Could you check a few things on this model? Use its own coordinates, in mm. Give positions to 0.01 mm unless a question says otherwise; leave off trailing zeros. Write each loop counter-clockwise with the first axis right and the second up, starting at its lowest first coordinate (ties: lowest second). Pieces come first, ordered by that corner, then holes. Notation, with made-up numbers: (34.5, 84.5) - (48.5, 84.5) arc R23 cw to (48.5, 109.5) - close; hole circle Ø7 at (-21, -4). An arc over 180 degrees is marked (long way). Answer as CSV lines item,"result". Start each with the question number.
Q1. Will these pins go through, and if not, where does the flat tip stop? pin 1 Ø2 at (x, z) = (15.5, -5) entering from -Y; pin 2 Ø1 at (x, y) = (35, 2) entering from +Z.
Q2. Imagine slicing it at D-D on z = 0. List the corners of the cut face in (x, y) for me, and give its area (3 significant figures).
Q3. Imagine slicing it at B-B on z = -19. List the corners of the cut face in (x, y) for me, and give its area (3 significant figures).
Q4. Imagine slicing it at A-A on y = 1.8. List the corners of the cut face in (x, z) for me, and give its area (3 significant figures).
Q5. If I drill on line 1 along X through (y, z) = (2.4, -19); line 2 along Z through (x, y) = (-9, 3.45); line 3 along Z through (x, y) = (-40, 2.45), over which ranges is the centre line in solid material (lowest first)?
Q6. Imagine slicing it at C-C on x = -40. List the corners of the cut face in (y, z) for me, and give its area (3 significant figures).
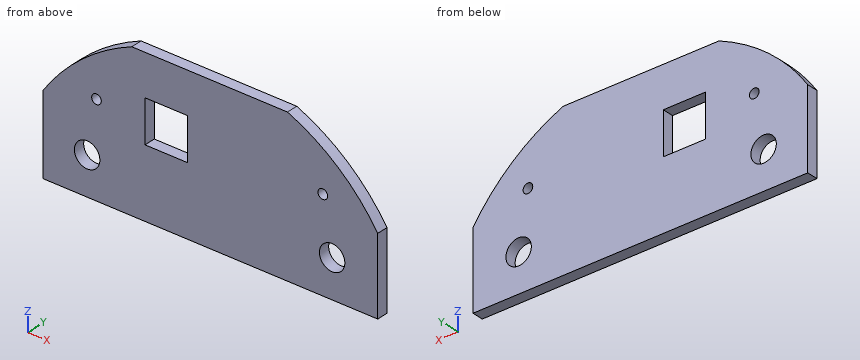
```python
from build123d import *

# Parameters (mm, degrees)
ESQUISSE1_W             = 63
ESQUISSE1_H             = 25
BOSS_EXTRU_1_DEPTH      = 4
D_GAGEMENT_M81_D        = 9
ESQUISSE5_R             = 96
ESQUISSE5_R_2           = 71
ENL_V_MAT_EXTRU_1_DEPTH = 68.845644546
ESQUISSE6_W             = 63
ESQUISSE6_H             = 25
BOSS_EXTRU_2_DEPTH      = 4
ESQUISSE7_W             = 15
ESQUISSE7_H             = 15
ENL_V_MAT_EXTRU_2_DEPTH = 68.845644546
D_GAGEMENT_M31_D        = 3.4


with BuildPart() as part:
    # Esquisse1 → Boss.-Extru.1 (new body)
    with BuildSketch(Plane(origin=(0, 0, 0), x_dir=(1, 0, 0), z_dir=(0, 1, 0))):
        Polygon((-58.901607841, 6.711500167), (-58.901607841, 32.486170288), (59.427941441, 32.486170288), (59.427941441, 7.487213227), (59.427941441, -21.450828615), (-58.901607841, -21.450828615), align=None)
        Rectangle(ESQUISSE1_W, ESQUISSE1_H, mode=Mode.SUBTRACT)
    extrude(amount=BOSS_EXTRU_1_DEPTH)

    # Dégagement M81 (through all)
    with Locations(Plane(origin=(0, 4, 0), x_dir=(1, 0, 0), z_dir=(0, 1, 0))):
        with Locations((-43.3, 19), (43.3, 19)):
            Hole(D_GAGEMENT_M81_D / 2)

    # Esquisse5 → Enlèv. mat.-Extru.1 (cut, through all)
    with BuildSketch(Plane(origin=(0, 4, 0), x_dir=(1, 0, 0), z_dir=(0, 1, 0))):
        with Locations((0, 44.002199903)):
            Circle(ESQUISSE5_R)
        with Locations((0, 44.002199903)):
            Circle(ESQUISSE5_R_2, mode=Mode.SUBTRACT)
    extrude(amount=-ENL_V_MAT_EXTRU_1_DEPTH, mode=Mode.SUBTRACT)

    # Esquisse6 → Boss.-Extru.2 (add)
    with BuildSketch(Plane(origin=(0, 4, 0), x_dir=(1, 0, 0), z_dir=(0, 1, 0))):
        Rectangle(ESQUISSE6_W, ESQUISSE6_H)
    extrude(amount=-BOSS_EXTRU_2_DEPTH)

    # Esquisse7 → Enlèv. mat.-Extru.2 (cut, through all)
    with BuildSketch(Plane(origin=(0, 4, 0), x_dir=(1, 0, 0), z_dir=(0, 1, 0))):
        with Locations((-15.335187954, 0.557700645)):
            Rectangle(ESQUISSE7_W, ESQUISSE7_H)
    extrude(amount=-ENL_V_MAT_EXTRU_2_DEPTH, mode=Mode.SUBTRACT)

    # Dégagement M31 (through all)
    with Locations(Plane(origin=(0, 4, 0), x_dir=(1, 0, 0), z_dir=(0, 1, 0))):
        with Locations((-40, 0), (40, 0)):
            Hole(D_GAGEMENT_M31_D / 2)


solid = part.part
```
Conclusion:
1,pin 1,"y = 0"
1,pin 2,"z = 18.05"
2,outline,"(-55.72, 0) - (-41.7, 0) - (-41.7, 4) - (-55.72, 4) - close; (-38.3, 0) - (-22.84, 0) - (-22.84, 4) - (-38.3, 4) - close; (-7.84, 0) - (38.3, 0) - (38.3, 4) - (-7.84, 4) - close; (41.7, 0) - (55.72, 0) - (55.72, 4) - (41.7, 4) - close"
2,area,"359 mm^2"
3,outline,"(-58.9, 0) - (-47.8, 0) - (-47.8, 4) - (-58.9, 4) - close; (-38.8, 0) - (38.8, 0) - (38.8, 4) - (-38.8, 4) - close; (47.8, 0) - (59.43, 0) - (59.43, 4) - (47.8, 4) - close"
3,area,"401 mm^2"
4,outline,"(-58.9, -32.49) - (59.43, -32.49) - (59.43, -5.15) arc R71 ccw to (27.51, 21.45) - (-27.51, 21.45) arc R71 ccw to (-58.9, -4.36) - close; hole circle Ø9 at (-43.3, -19); hole circle Ø3.4 at (-40, 0); hole (-22.84, -8.06) - (-7.84, -8.06) - (-7.84, 6.94) - (-22.84, 6.94) - close; hole circle Ø3.4 at (40, 0); hole circle Ø9 at (43.3, -19)"
4,area,"5,350 mm^2"
5,line 1,"-58.9 to -47.8, -38.8 to 38.8, 47.8 to 59.43"
5,line 2,"-32.49 to -8.06, 6.94 to 21.45"
5,line 3,"-32.49 to -22.06, -15.94 to -1.7, 1.7 to 14.66"
6,outline,"(0, -32.49) - (4, -32.49) - (4, -22.06) - (0, -22.06) - close; (0, -15.94) - (4, -15.94) - (4, -1.7) - (0, -1.7) - close; (0, 1.7) - (4, 1.7) - (4, 14.66) - (0, 14.66) - close"
6,area,"151 mm^2"
